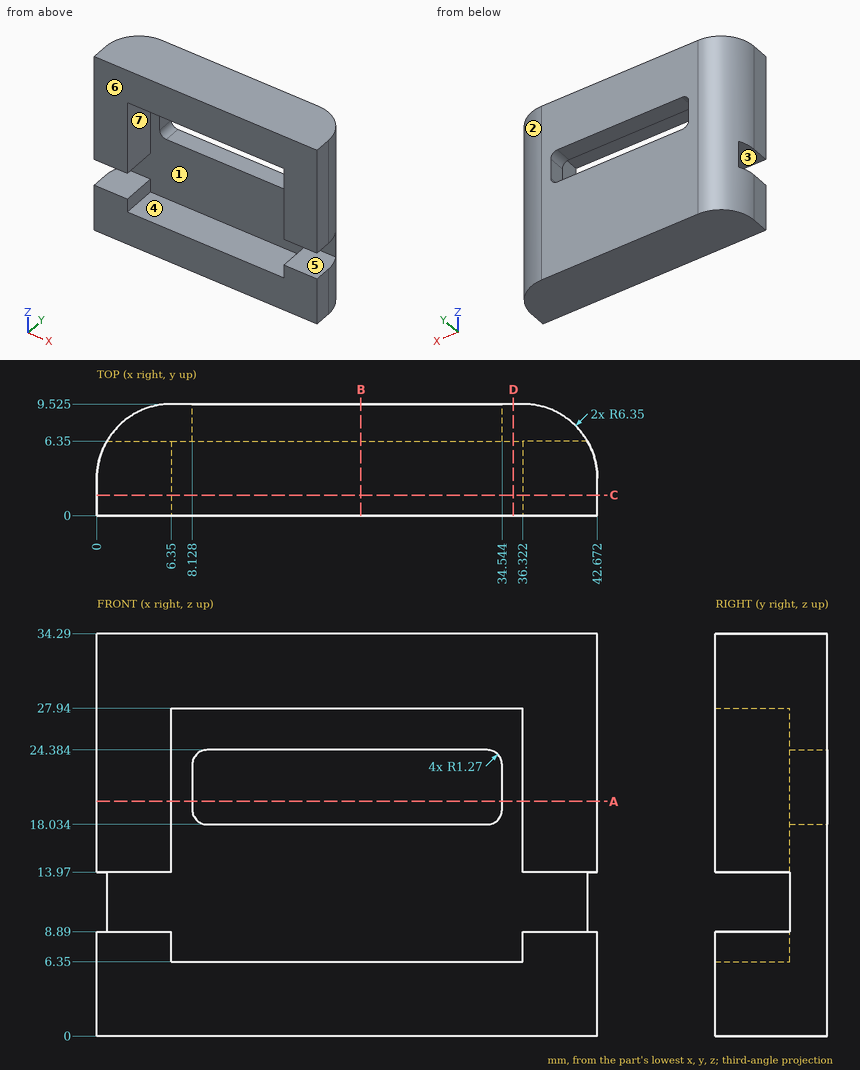
Geometry: see drawing. Coordinates: mm, zero at the bounding-box minimum. A direction names the side the tool comes from. Round coordinates to 2 decimals unless told otherwise and drop trailing zeros. Write each loop counter-clockwise with the first axis right and the second up, starting at its lowest first coordinate (ties: lowest second). Pieces come first, ordered by that corner, then holes. Notation, with made-up numbers: M 81.25,17 L 119.25,17 A14 ccw 119.25,39 Z; hole C 15,38.25 d1. An arc over 180 degrees is marked long. Answer as a JSON object with one key per item and string values. Group by question number.
(1) Section query A-A on z = 20. Output: boundary loops of the cut face in (x, y) (3 decimals), then the cut area to 3 significant figures.
(2) First-contact query: pin 1 (1.5 mm diameter, centred on x = 30, y = 8.5, fed in from -Z); pin 2 (1 mm diameter, centred on y = 8, z = 20.5, fed in from +X); pin 3 (6.5 mm diameter, centred on x = 26, z = 19.5, fed in from -Y); pin 4 (3 mm diameter, centred on x = 11.5, z = 22, fed in from -Y). Flat tips, straight axial feed; report the tip coordinate or a pass-through.
(3) Section query C-C on y = 1.75. Output: boundary loops of the cut face in (x, z), then the cut area to 3 significant figures.
(4) Mould query, pull axis X, two halves, no side actions, for the marked faces 1, 2, 3 and 4. Classes: +X half, -X half, draft (parallel to the pull), parting line (faces both ways), or undercut.
(5) Ray query, line 1 (Z direction, x = 28.5, y = 5.25); line 2 (X direction, y = 3.25, z = 27); line 3 (Z direction, x = 39.5, y = 0.75). Return the intervals inside material, ascending. Write a range as [from, to].
(6) Section query B-B on x = 22.5. Output: boundary loops of the cut face in (y, z) (3 decimals).
(7) Section query D-D on x = 35.5. Output: boundary loops of the cut face in (y, z) (3 decimals).
(8) Reachability of the marked faces 5, 6 and 7 from +Z, -Z, +X, -X, +Y, -Y: full face, straight path, thin tool, end or side. Return the list, or none.
Computed values:
{
 "1": {"outline": "M 0,0 L 6.35,0 L 6.35,6.35 L 8.128,6.35 L 8.128,9.525 L 6.35,9.525 A6.35 ccw 0,3.175 Z; M 34.544,6.35 L 36.322,6.35 L 36.322,0 L 42.672,0 L 42.672,3.175 A6.35 ccw 36.322,9.525 L 34.544,9.525 Z", "area": "115 mm^2"},
 "2": {"pin 1": "z = 0", "pin 2": "x = 40.97", "pin 3": "y = 6.35", "pin 4": "through"},
 "3": {"outline": "M 0,0 L 42.67,0 L 42.67,8.89 L 36.32,8.89 L 36.32,6.35 L 6.35,6.35 L 6.35,8.89 L 0,8.89 Z; M 0,13.97 L 6.35,13.97 L 6.35,27.94 L 36.32,27.94 L 36.32,13.97 L 42.67,13.97 L 42.67,34.29 L 0,34.29 Z", "area": "752 mm^2"},
 "4": {"face 1": "undercut", "face 2": "+X half", "face 3": "draft", "face 4": "undercut"},
 "5": {"line 1": "[0, 6.35], [27.94, 34.29]", "line 2": "[0, 6.35], [36.32, 42.67]", "line 3": "[0, 8.89], [13.97, 34.29]"},
 "6": {"outline": "M 0,0 L 9.525,0 L 9.525,18.034 L 6.35,18.034 L 6.35,6.35 L 0,6.35 Z; M 0,27.94 L 6.35,27.94 L 6.35,24.384 L 9.525,24.384 L 9.525,34.29 L 0,34.29 Z"},
 "7": {"outline": "M 0,0 L 9.525,0 L 9.525,34.29 L 0,34.29 L 0,27.94 L 6.35,27.94 L 6.35,6.35 L 0,6.35 Z"},
 "8": {"face 5": "+X, -X, -Y", "face 6": "+Z, -Z, +X, -X, -Y", "face 7": "-Y"}
}
